```python
from build123d import *

# Parameters (mm, degrees)
F1_DEPTH      = 38.1
F1_DEPTH_BACK = 38.1


with BuildPart() as f1:
    # F0 (on Top) → F1 (new body, two sides)
    with BuildSketch(Plane.XY) as f1_sk:
        with BuildLine():
            ThreePointArc((-90.6969597738, 13.086746717), (-76.7539676292, 16.2972540142), (-70.5542587543, 29.1921366006))
            ThreePointArc((-70.5542587543, 29.1921366006), (-70.7418172824, 31.673669272), (-71.3002314253, 34.0988200397))
            ThreePointArc((-71.3002314253, 34.0988200397), (-83.4315577445, 45.2975264864), (-99.1955851313, 40.3908427907))
            ThreePointArc((-99.1955851313, 40.3908427907), (-102.828286017, 24.2854529488), (-90.6969597738, 13.086746717))
        make_face()
        with BuildLine():
            ThreePointArc((-77.3292507738, 30.1186681005), (-77.2962629506, 29.6559242455), (-77.2852587543, 29.1921366006))
            ThreePointArc((-77.2852587543, 29.1921366006), (-77.3859317475, 27.7925554665), (-77.6858779078, 26.4217911893))
            ThreePointArc((-77.6858779078, 26.4217911893), (-76.7965239356, 25.6970936215), (-76.4622244556, 24.5996507254))
            ThreePointArc((-76.4622244556, 24.5996507254), (-77.5033356386, 22.8632918247), (-79.5254118898, 22.9636031493))
            ThreePointArc((-79.5254118898, 22.9636031493), (-80.8453813803, 21.6453223583), (-82.3916720877, 20.6016898809))
            ThreePointArc((-82.3916720877, 20.6016898809), (-82.2770283841, 20.2284516132), (-82.2383060109, 19.8399280476))
            ThreePointArc((-82.2383060109, 19.8399280476), (-84.0144862482, 17.8808452625), (-86.1377272544, 19.4571286201))
            ThreePointArc((-86.1377272544, 19.4571286201), (-88.0032519189, 19.458322711), (-89.8346041656, 19.8137557541))
            ThreePointArc((-89.8346041656, 19.8137557541), (-92.5812060719, 18.82068306), (-93.2927922056, 21.6532897362))
            ThreePointArc((-93.2927922056, 21.6532897362), (-94.6110729966, 22.9732592267), (-95.6547054739, 24.5195499341))
            ThreePointArc((-95.6547054739, 24.5195499341), (-98.2990547433, 25.759482331), (-96.7992667347, 28.2656051007))
            ThreePointArc((-96.7992667347, 28.2656051007), (-96.7980726438, 30.1311297652), (-96.4426396008, 31.9624820119))
            ThreePointArc((-96.4426396008, 31.9624820119), (-97.4357122948, 34.7090839182), (-94.6031056187, 35.420670052))
            ThreePointArc((-94.6031056187, 35.420670052), (-93.2831361282, 36.7389508429), (-91.7368454208, 37.7825833203))
            ThreePointArc((-91.7368454208, 37.7825833203), (-90.4969130238, 40.4269325897), (-87.9907902541, 38.9271445811))
            ThreePointArc((-87.9907902541, 38.9271445811), (-86.1252655897, 38.9259504902), (-84.2939133429, 38.5705174471))
            ThreePointArc((-84.2939133429, 38.5705174471), (-82.0922279233, 39.7572344826), (-80.503272879, 37.8256708993))
            ThreePointArc((-80.503272879, 37.8256708993), (-80.5882188045, 37.2536426673), (-80.8357253029, 36.7309834651))
            ThreePointArc((-80.8357253029, 36.7309834651), (-79.517444512, 35.4110139746), (-78.4738120346, 33.8647232672))
            ThreePointArc((-78.4738120346, 33.8647232672), (-76.622219003, 33.688875838), (-75.7435502012, 32.0495893439))
            ThreePointArc((-75.7435502012, 32.0495893439), (-76.1907788706, 30.8002992301), (-77.3292507738, 30.1186681005))
        make_face(mode=Mode.SUBTRACT)
        with BuildLine():
            ThreePointArc((-71.3002314253, 34.0988200397), (-70.7418172824, 31.673669272), (-70.5542587543, 29.1921366006))
            ThreePointArc((-70.5542587543, 29.1921366006), (-76.7539676292, 16.2972540142), (-90.6969597738, 13.086746717))
            ThreePointArc((-90.6969597738, 13.086746717), (-71.5368890892, 3.9232487058), (-58.2455134206, -12.6422979885))
            ThreePointArc((-58.2455134206, -12.6422979885), (-49.7371002236, -5.2654204228), (-43.0629257789, 3.804685047))
            ThreePointArc((-43.0629257789, 3.804685047), (-60.6365657041, 15.7313428229), (-71.3002314253, 34.0988200397))
        make_face()
        with BuildLine():
            ThreePointArc((-99.1955851313, 40.3908427907), (-83.4315577445, 45.2975264864), (-71.3002314253, 34.0988200397))
            ThreePointArc((-71.3002314253, 34.0988200397), (-72.9444447549, 55.2736770618), (-65.2439483139, 75.0671194593))
            ThreePointArc((-65.2439483139, 75.0671194593), (-75.8867182849, 78.747182651), (-87.0787472591, 79.9921345345))
            ThreePointArc((-87.0787472591, 79.9921345345), (-88.6207159571, 58.8095868891), (-99.1955851313, 40.3908427907))
        make_face()
        with BuildLine():
            ThreePointArc((-131.0511032248, 3.7795902204), (-111.9354945769, 13.0354799606), (-90.6969597738, 13.086746717))
            ThreePointArc((-90.6969597738, 13.086746717), (-102.828286017, 24.2854529488), (-99.1955851313, 40.3908427907))
            ThreePointArc((-99.1955851313, 40.3908427907), (-116.7114425044, 28.3794839343), (-137.7033145282, 25.151588331))
            ThreePointArc((-137.7033145282, 25.151588331), (-135.5689577543, 14.0946475737), (-131.0511032248, 3.7795902204))
        make_face()
        with BuildLine():
            ThreePointArc((-77.6858779078, 26.4217911893), (-77.3859317475, 27.7925554665), (-77.2852587543, 29.1921366006))
            ThreePointArc((-77.2852587543, 29.1921366006), (-77.2962629506, 29.6559242455), (-77.3292507738, 30.1186681005))
            ThreePointArc((-77.3292507738, 30.1186681005), (-79.5946376372, 31.4743878177), (-78.4738120346, 33.8647232672))
            ThreePointArc((-78.4738120346, 33.8647232672), (-79.517444512, 35.4110139746), (-80.8357253029, 36.7309834651))
            ThreePointArc((-80.8357253029, 36.7309834651), (-83.3962343215, 36.0877516573), (-84.2939133429, 38.5705174471))
            ThreePointArc((-84.2939133429, 38.5705174471), (-86.1252655897, 38.9259504902), (-87.9907902541, 38.9271445811))
            ThreePointArc((-87.9907902541, 38.9271445811), (-87.9626287125, 38.7366649164), (-87.9532114976, 38.5443451537))
            ThreePointArc((-87.9532114976, 38.5443451537), (-89.5331879319, 36.6145675269), (-91.7368454208, 37.7825833203))
            ThreePointArc((-91.7368454208, 37.7825833203), (-93.2831361282, 36.7389508429), (-94.6031056187, 35.420670052))
            ThreePointArc((-94.6031056187, 35.420670052), (-93.9614341522, 34.7120112928), (-93.7292930529, 33.7846224758))
            ThreePointArc((-93.7292930529, 33.7846224758), (-94.6003501568, 32.1504219558), (-96.4426396008, 31.9624820119))
            ThreePointArc((-96.4426396008, 31.9624820119), (-96.7980726438, 30.1311297652), (-96.7992667347, 28.2656051007))
            ThreePointArc((-96.7992667347, 28.2656051007), (-95.1671771935, 27.8559551879), (-94.4479673073, 26.3346838573))
            ThreePointArc((-94.4479673073, 26.3346838573), (-94.7771808133, 25.2448526591), (-95.6547054739, 24.5195499341))
            ThreePointArc((-95.6547054739, 24.5195499341), (-94.6110729966, 22.9732592267), (-93.2927922056, 21.6532897362))
            ThreePointArc((-93.2927922056, 21.6532897362), (-91.0847163975, 22.4421563765), (-89.6882446295, 20.558602302))
            ThreePointArc((-89.6882446295, 20.558602302), (-89.7251810461, 20.1790573462), (-89.8346041656, 19.8137557541))
            ThreePointArc((-89.8346041656, 19.8137557541), (-88.0032519189, 19.458322711), (-86.1377272544, 19.4571286201))
            ThreePointArc((-86.1377272544, 19.4571286201), (-84.7820075372, 21.7225154836), (-82.3916720877, 20.6016898809))
            ThreePointArc((-82.3916720877, 20.6016898809), (-80.8453813803, 21.6453223583), (-79.5254118898, 22.9636031493))
            ThreePointArc((-79.5254118898, 22.9636031493), (-80.1686436975, 25.5241121678), (-77.6858779078, 26.4217911893))
        make_face()
    extrude(amount=F1_DEPTH)
    extrude(f1_sk.sketch, amount=-F1_DEPTH_BACK)


solid = f1.part
```
Model file for the job. Use its own axes, mm. Round coordinates to 2 decimals unless told otherwise and drop trailing zeros. Write each loop counter-clockwise with the first axis right and the second up, starting at its lowest first coordinate (ties: lowest second). Pieces come first, ordered by that corner, then holes. Notation, with made-up numbers: (-6, 28) - (51, 28) arc R35 cw to (51, 66) - close; hole circle Ø2 at (71, 70). An arc over 180 degrees is marked (long way). Use CSV: the item, a comma, the result in double quotes. Start each with the question number.
Item 1: Band-saw the part on C-C (x = -103.5). Write the cut outline in (y, z).
Item 2: Band-saw the part on A-A (z = 28). State how many separate pieces and enclosed holes the cut face has, and give its area (3 significant figures).
Item 3: Drill centre lines: L1, parallel to X at y = 32.5, z = -16; L2, parallel to Y at x = -79.5, z = 24; L3, parallel to Y at x = -114, z = 16. Where is each one in solid material? Low to high. Write a range as [from, to].
Item 4: Pin check, flat tips, straight feed: P1, Ø4.5, axis at x = -96.42, y = 26.33, coming from the +Z side; P2, Ø8, axis at y = 9, z = 2.5, coming from the -X side; P3, Ø2.5, axis at x = -91.66, y = 20.56, coming from the -Z side; P4, Ø1, axis at x = -102.5, z = -13, coming from the -Y side. Stop position of each tip, or through.
Item 5: Two-plate mould, pull along Y, no slides. Class faces 1 (the face through (-98.792, 40.834, 0.533)), 2 (the face through (-87, 30, 38.1)), 3 (the face through (-75.73, 78.71, 0.53)), 4 (the face through (-135.6, 14.2, 0.5)): released by +Y, released by -Y, zero draft, split by the parting line, or undercut.
Item 6: Band-saw the part on B-B (y = -3). Write the cut outline in (x, z).
Checked values:
1,outline,"(14.2, -38.1) - (36.28, -38.1) - (36.28, 38.1) - (14.2, 38.1) - close"
2,separate pieces,"1"
2,enclosed holes,"8"
2,area,"2,680 mm²"
3,L1,"x = [-108.64, -97.19], [-94.21, -79.63], [-75.8, -70.77]"
3,L2,"y = [9.04, 22.95], [26.25, 31.23], [32.87, 79.43]"
3,L3,"y = [12.51, 29.55]"
4,P1,"stops at z = 38.1"
4,P2,"stops at x = -135.21"
4,P3,"passes through"
4,P4,"stops at y = 14.22"
5,face 1,"undercut"
5,face 2,"zero draft"
5,face 3,"released by +Y"
5,face 4,"released by -Y"
6,outline,"(-64.46, -38.1) - (-47.77, -38.1) - (-47.77, 38.1) - (-64.46, 38.1) - close"
